Source: CAD feature listing. Evaluate the final solid. Frame: model axes, mm. A direction names the side the tool comes from. Give positions to 0.01 mm unless a question says otherwise; leave off trailing zeros. Order: outer loops, then holes, each group sorted by start corner. A loop starts at its lowest first (then second) coordinate and runs counter-clockwise, first axis right, second up. Notation, with made-up numbers: M 68.5,-9.5 L 103.5,-9.5 A8 ccw 103.5,-1.5 Z; hole C 42.25,35 d6. An arc over 180 degrees is marked long. Answer in a Markdown table with one row per item. Add a question column.
(1) Pin query (flat end, axial travel): P1, Ø1, axis at y = 36, z = -9, coming from the +X side; P2, Ø11, axis at y = 14.5, z = -9, coming from the -X side; P3, Ø1.8, axis at x = -62.8, z = 15.5, coming from the -Y side; P4, Ø2, axis at y = 80, z = -6.5, coming from the +X side. Return the tip coordinate at first contact, or that it passes through.
(2) Section query C-C, the plane x = 10. Return loops of the section in (y, z), plus the area to 3 significant figures.
(3) Section query B-B, the plane z = -6. Return loops of the section in (x, y), plus the area to 3 significant figures.
(4) Section query D-D, the plane y = 38.5. Return loops of the section in (x, z).
(5) Section query A-A, the plane y = 66. Return loops of the section in (x, z).
(6) Mould query, pull axis Z, two halves, no side actions, for faces 5 (the face through (0, 15, 21.15)), 6 (the face through (-26.15, 15, 0)), 7 (the face through (100, 5, 0)). Classes: pulls with the +Z half, pulls with the -Z half, needs draft (parallel to the pull), parting line crosses it, or undercut.
(7) Material intervals for line 1 along X through (y, z) = (11.55, 0); line 2 along X through (y, z) = (13, -15.5); line 3 along X through (y, z) = (4.25, 15.5), sorted ascending.
(8) Set-up query: faces 1 (the face through (0, 15, -21.15)), 2 (the face through (-77.638, 44, 0)), 3 (the face through (-68.45, 40, 0)), 4 (the face through (100, 8, -10)). Return all of +Z, -Z, +X, -X, +Y, -Y with unobstructed straight access to the full face (end or side cutting, diameter ignored); none if empty.
from build123d import *

# Parameters (mm, degrees)
SKETCH2_R           = 1.5
BOSS_EXTRUDE1_DEPTH = 10
SKETCH3_W           = 25
SKETCH3_H           = 20
CUT_EXTRUDE1_DEPTH  = 5
SKETCH5_R           = 18
SKETCH5_R_2         = 17
BOSS_EXTRUDE2_DEPTH = 2
SKETCH2_3_W         = 42.3
SKETCH2_3_H         = 42.3
SKETCH2_3_R         = 1.5
BOSS_EXTRUDE3_DEPTH = 20
SKETCH8_W           = 40
SKETCH8_H           = 60
BOSS_EXTRUDE4_DEPTH = 10
SKETCH9_W           = 42.3
SKETCH9_H           = 42.3
SKETCH9_R           = 1.5
BOSS_EXTRUDE5_DEPTH = 10
CUT_EXTRUDE3_START  = -10
SKETCH9_3_R         = 1.5
CUT_EXTRUDE3_DEPTH  = 10
SKETCH10_W          = 9.18782392
SKETCH10_H          = 60
BOSS_EXTRUDE6_DEPTH = 80
BOSS_EXTRUDE7_DEPTH = 8.75
BOSS_EXTRUDE9_DEPTH = 10
SKETCH16_W          = 42.5
SKETCH16_H          = 10
CUT_EXTRUDE5_DEPTH  = 9.18782392


with BuildPart() as part:
    # Sketch2 → Boss-Extrude1 (new body)
    with BuildSketch(Plane(origin=(0, 0, 0), x_dir=(1, 0, 0), z_dir=(0, 1, 0))):
        with BuildLine():
            Line((-37.63782392, -30), (100, -30))
            ThreePointArc((100, -30), (130, 0), (100, 30))
            Line((100, 30), (-37.63782392, 30))
            Line((-37.63782392, 30), (-37.63782392, -30))
        make_face()
        with Locations(Location((-15.5, 15.5, 0), (0, 0, 270))):
            Circle(SKETCH2_R, mode=Mode.SUBTRACT)
        with Locations(Location((15.5, -15.5, 0), (0, 0, 270))):
            Circle(SKETCH2_R, mode=Mode.SUBTRACT)
        with Locations(Location((-15.5, -15.5, 0), (0, 0, 270))):
            Circle(SKETCH2_R, mode=Mode.SUBTRACT)
        with Locations(Location((15.5, 15.5, 0), (0, 0, 270))):
            Circle(SKETCH2_R, mode=Mode.SUBTRACT)
    extrude(amount=BOSS_EXTRUDE1_DEPTH)

    # Sketch3 → Cut-Extrude1 (cut)
    with BuildSketch(Plane(origin=(0, 10, 0), x_dir=(1, 0, 0), z_dir=(0, 1, 0))):
        with Locations((100, 0)):
            Rectangle(SKETCH3_W, SKETCH3_H)
    extrude(amount=-CUT_EXTRUDE1_DEPTH, mode=Mode.SUBTRACT)

    # Sketch5 → Boss-Extrude2 (add)
    with BuildSketch(Plane(origin=(0, 10, 0), x_dir=(1, 0, 0), z_dir=(0, 1, 0))):
        with Locations(Location((100, 0, 0), (0, 0, 270))):
            Circle(SKETCH5_R)
        with Locations(Location((100, 0, 0), (0, 0, 270))):
            Circle(SKETCH5_R_2, mode=Mode.SUBTRACT)
    extrude(amount=BOSS_EXTRUDE2_DEPTH)

    # Sketch2<3> → Boss-Extrude3 (add)
    with BuildSketch(Plane(origin=(0, 0, 0), x_dir=(1, 0, 0), z_dir=(0, 1, 0))):
        Rectangle(SKETCH2_3_W, SKETCH2_3_H)
        with Locations(Location((-15.5, -15.5, 0), (0, 0, 270))):
            Circle(SKETCH2_3_R, mode=Mode.SUBTRACT)
        with Locations(Location((15.5, -15.5, 0), (0, 0, 270))):
            Circle(SKETCH2_3_R, mode=Mode.SUBTRACT)
        with Locations(Location((15.5, 15.5, 0), (0, 0, 270))):
            Circle(SKETCH2_3_R, mode=Mode.SUBTRACT)
        with Locations(Location((-15.5, 15.5, 0), (0, 0, 270))):
            Circle(SKETCH2_3_R, mode=Mode.SUBTRACT)
    extrude(amount=BOSS_EXTRUDE3_DEPTH)

    # Sketch8 → Boss-Extrude4 (add)
    with BuildSketch(Plane.XZ):
        with Locations((-57.63782392, 0)):
            Rectangle(SKETCH8_W, SKETCH8_H)
    extrude(amount=-BOSS_EXTRUDE4_DEPTH)

    # Sketch9 → Boss-Extrude5 (add)
    with BuildSketch(Plane(origin=(0, 10, 0), x_dir=(1, 0, 0), z_dir=(0, 1, 0))):
        with Locations((-47.3, 0)):
            Rectangle(SKETCH9_W, SKETCH9_H)
        with Locations(Location((-31.8, 15.5, 0), (0, 0, 270))):
            Circle(SKETCH9_R, mode=Mode.SUBTRACT)
        with Locations(Location((-31.8, -15.5, 0), (0, 0, 270))):
            Circle(SKETCH9_R, mode=Mode.SUBTRACT)
        with Locations(Location((-62.8, -15.5, 0), (0, 0, 270))):
            Circle(SKETCH9_R, mode=Mode.SUBTRACT)
        with Locations(Location((-62.8, 15.5, 0), (0, 0, 270))):
            Circle(SKETCH9_R, mode=Mode.SUBTRACT)
    extrude(amount=BOSS_EXTRUDE5_DEPTH)

    # Sketch9<3> → Cut-Extrude3 (cut)
    with BuildSketch(Plane(origin=(0, 10, 0), x_dir=(1, 0, 0), z_dir=(0, 1, 0)).offset(CUT_EXTRUDE3_START)):
        with Locations(Location((-62.8, -15.5, 0), (0, 0, 270))):
            Circle(SKETCH9_3_R)
        with Locations(Location((-31.8, -15.5, 0), (0, 0, 270))):
            Circle(SKETCH9_3_R)
        with Locations(Location((-31.8, 15.5, 0), (0, 0, 270))):
            Circle(SKETCH9_3_R)
        with Locations(Location((-62.8, 15.5, 0), (0, 0, 270))):
            Circle(SKETCH9_3_R)
    extrude(amount=CUT_EXTRUDE3_DEPTH, mode=Mode.SUBTRACT)

    # Sketch10 → Boss-Extrude6 (add)
    with BuildSketch(Plane(origin=(0, 10, 0), x_dir=(1, 0, 0), z_dir=(0, 1, 0))):
        with Locations((-73.04391196, 0)):
            Rectangle(SKETCH10_W, SKETCH10_H)
    extrude(amount=BOSS_EXTRUDE6_DEPTH)

    # Sketch13 → Boss-Extrude7 (add)
    with BuildSketch(Plane.XY.offset(30)):
        Polygon((-68.45, 90), (-26.15, 10), (-68.45, 10), align=None)
    boss_extrude7 = extrude(amount=-BOSS_EXTRUDE7_DEPTH)

    # Mirror2: Boss-Extrude7 across plane
    add(boss_extrude7.mirror(Plane.XY))

    # Sketch11 → Boss-Extrude9 (add)
    with BuildSketch(Plane.ZY.offset(77.63782392)):
        with BuildLine():
            ThreePointArc((-15, 80), (-23.535533906, 83.535533906), (-20, 75))
            Line((-20, 75), (-20, 80))
            Line((-20, 80), (-15, 80))
        make_face()
        with BuildLine():
            Line((-20, 80), (-20, 75))
            ThreePointArc((-20, 75), (-16.464466094, 76.464466094), (-15, 80))
            Line((-15, 80), (-20, 80))
        make_face()
        with BuildLine():
            ThreePointArc((15, 80), (16.464466094, 76.464466094), (20, 75))
            Line((20, 75), (20, 80))
            Line((20, 80), (15, 80))
        make_face()
        with BuildLine():
            Line((20, 80), (20, 75))
            ThreePointArc((20, 75), (23.535533906, 76.464466094), (25, 80))
            ThreePointArc((25, 80), (20, 85), (15, 80))
            Line((15, 80), (20, 80))
        make_face()
        with BuildLine():
            ThreePointArc((20, 15), (16.464466094, 13.535533906), (15, 10))
            Line((15, 10), (20, 10))
            Line((20, 10), (20, 15))
        make_face()
        with BuildLine():
            Line((20, 10), (15, 10))
            ThreePointArc((15, 10), (20, 5), (25, 10))
            ThreePointArc((25, 10), (23.535533906, 13.535533906), (20, 15))
            Line((20, 15), (20, 10))
        make_face()
        with BuildLine():
            Line((-20, 15), (-20, 10))
            Line((-20, 10), (-15, 10))
            ThreePointArc((-15, 10), (-16.464466094, 13.535533906), (-20, 15))
        make_face()
        with BuildLine():
            Line((-15, 10), (-20, 10))
            Line((-20, 10), (-20, 15))
            ThreePointArc((-20, 15), (-23.535533906, 6.464466094), (-15, 10))
        make_face()
    extrude(amount=BOSS_EXTRUDE9_DEPTH)

    # Sketch16 → Cut-Extrude5 (cut)
    with BuildSketch(Plane(origin=(-68.45, 0, 0), x_dir=(0, 0, -1), z_dir=(1, 0, 0))):
        with Locations((0, 65)):
            Rectangle(SKETCH16_W, SKETCH16_H)
    extrude(amount=-CUT_EXTRUDE5_DEPTH, mode=Mode.SUBTRACT)


solid = part.part
Values follow:
| question | item | result |
|---|---|---|
| 1 | P1 | stops at x = -68.45 |
| 1 | P2 | stops at x = -77.64 |
| 1 | P3 | passes through |
| 1 | P4 | stops at x = -68.45 |
| 2 | outline | M 0,-30 L 10,-30 L 10,-21.15 L 20,-21.15 L 20,21.15 L 10,21.15 L 10,30 L 0,30 Z |
| 2 | area | 1,020 mm² |
| 3 | outline | M -77.64,0 L 129.39,0 L 129.39,10 L 116.97,10 L 116.97,12 L 115.91,12 L 115.91,10 L 112.5,10 L 112.5,5 L 87.5,5 L 87.5,10 L 84.09,10 L 84.09,12 L 83.03,12 L 83.03,10 L 21.15,10 L 21.15,20 L -21.15,20 L -21.15,10 L -26.15,10 L -26.15,20 L -68.45,20 L -68.45,60 L -77.64,60 Z; M -77.64,70 L -68.45,70 L -68.45,90 L -77.64,90 Z |
| 3 | area | 3,440 mm² |
| 4 | outline | M -77.64,-30 L -41.22,-30 L -41.22,-21.25 L -68.45,-21.25 L -68.45,21.25 L -41.22,21.25 L -41.22,30 L -77.64,30 Z |
| 5 | outline | M -77.64,-30 L -55.76,-30 L -55.76,-21.25 L -77.64,-21.25 Z; M -77.64,21.25 L -55.76,21.25 L -55.76,30 L -77.64,30 Z |
| 6 | face 5 | pulls with the +Z half |
| 6 | face 6 | needs draft |
| 6 | face 7 | undercut |
| 7 | line 1 | x = -77.64 to -26.15, -21.15 to 21.15, 82 to 83, 117 to 118 |
| 7 | line 2 | x = -77.64 to -64.3, -61.3 to -33.3, -30.3 to -26.15, -21.15 to -17, -14 to 14, 17 to 21.15 |
| 7 | line 3 | x = -77.64 to -64.3, -61.3 to -33.3, -30.3 to -17, -14 to 14, 17 to 125.69 |
| 8 | face 1 | -Z, +X, +Y |
| 8 | face 2 | -X |
| 8 | face 3 | +X, +Y |
| 8 | face 4 | +Y |
